```python
from build123d import *

# Parameters (mm, degrees)
F0_R      = 16.75
F1_DEPTH  = 6.2
F2_R      = 23.65
F3_DEPTH  = 2.2
F5_D      = 2
F6_R      = 16
F7_DEPTH  = 3.9
F8_R      = 12.5
F9_DEPTH  = 4.5
F11_D     = 1
F11_DEPTH = 4
F11_TIP   = 0.3004303095
F12_R     = 7.2
F13_DEPTH = 6.6
F15_D     = 3
F15_DEPTH = 1
F15_TIP   = 0.9012909285


with BuildPart() as f1:
    # F0 (on Top) → F1 (new body)
    with BuildSketch(Plane.XY):
        Circle(F0_R)
    extrude(amount=F1_DEPTH)

    # F2 (on face) → F3 (join)
    with BuildSketch(Plane.XY.offset(6.2)):
        Circle(F2_R)
    extrude(amount=F3_DEPTH)

    # F5 (through all)
    with Locations(Plane.XY.offset(8.4)):
        with Locations((0, 20.65), (17.8834245881, -10.325), (-17.8834245881, -10.325)):
            Hole(F5_D / 2)

    # F6 (on face) → F7 (join)
    with BuildSketch(Plane.XY.offset(8.4)):
        Circle(F6_R)
    extrude(amount=F7_DEPTH)

    # F8 (on face) → F9 (join)
    with BuildSketch(Plane.XY.offset(12.3)):
        Circle(F8_R)
    extrude(amount=F9_DEPTH)

    # F11
    with Locations(Plane.XY.offset(16.8)):
        with Locations((-8.6602540378, 5), (0, 10), (8.6602540378, 5), (8.6602540378, -5), (0, -10), (-8.6602540378, -5)):
            Hole(F11_D / 2, depth=F11_DEPTH)
            with Locations((0, 0, -(F11_DEPTH + F11_TIP / 2))):  # 118° drill point
                Cone(0, F11_D / 2, F11_TIP, mode=Mode.SUBTRACT)

    # F12 (on face) → F13 (join)
    with BuildSketch(Plane.XY.offset(16.8)):
        Circle(F12_R)
    extrude(amount=F13_DEPTH)

    # F15
    with Locations(Plane.XY.offset(23.4)):
        with Locations((0, 0)):
            Hole(F15_D / 2, depth=F15_DEPTH)
            with Locations((0, 0, -(F15_DEPTH + F15_TIP / 2))):  # 118° drill point
                Cone(0, F15_D / 2, F15_TIP, mode=Mode.SUBTRACT)


solid = f1.part
```
Design review of the part built by this model. Coordinates are the model's own, in mm. A direction names the side the tool comes from. Give positions to 0.01 mm unless a question says otherwise; leave off trailing zeros. Order: outer loops, then holes, each group sorted by start corner. A loop starts at its lowest first (then second) coordinate and runs counter-clockwise, first axis right, second up. Notation, with made-up numbers: (9, 86.25) - (42, 86.25) arc R26 ccw to (42, 125.25) - close; hole circle Ø10 at (21.5, 59.5). An arc over 180 degrees is marked (long way). Use a Markdown table: item, result. Add a question column.
(1) Add section D-D on y = -8.5. Give the boundary of the cut face in (x, z).
(2) Add section A-A on y = 20.65. Give the boundary of the cut face in (x, z), then the cut area to 3 significant figures.
(3) Mouldability with a two-part tool opening along X and no side actions: class faces 1 (the face through (0.13, 21.64, 7.28)), 2 (the face through (-5.127, -23.088, 7.285)), 3 (the face through (0, 0, 0)), 4 (the face through (-17.09, -10.933, 7.285)) as +X half, -X half, draft (parallel to the pull), parting line (faces both ways), or undercut.
(4) Wall thickness on probe 1 along X at (y, z) = (-5, 14.9); probe 2 along Y at (x, z) = (0, 11.25); probe 3 along Z at (x, y) = (15.5, 11): over which ranges is each line inside the solid? List them lowest first. Write a range as [from, to].
(5) Add section C-C on x = 14. Give the boundary of the cut face in (y, z), then the cut area to 3 significant figures.
(6) Machinability: for faces 5 (the face through (18.7, -10.9, 7.3)), 6 (the face through (-3.63, -16.35, 3.06)), 7 (the face through (4.9, -15.4, 8.4)), which of the approach directions +Z, -Z, +X, -X, +Y, -Y give a long, thin tool a straight path to every point of the face, cutting with its end or side? Answer none if there is none.
(7) Add section B-B on y = -3.5. Give the boundary of the cut face in (x, z).
(8) Clearance check with flat-ended pins moving along their axes: P1, Ø3, axis at x = 4.5, y = 16, coming from the +Z side; P2, Ø5, axis at y = -15, z = 17.5, coming from the +X side; P3, Ø12, axis at x = -3, z = 6, coming from the -Y side; P4, Ø2.5, axis at x = -17.88, y = -10.32, coming from the -Z side. State where each tip first meets the part, or that it passes through.
Report:
| question | item | result |
|---|---|---|
| 1 | outline | (-22.07, 6.2) - (-14.43, 6.2) - (-14.43, 0) - (14.43, 0) - (14.43, 6.2) - (22.07, 6.2) - (22.07, 8.4) - (13.56, 8.4) - (13.56, 12.3) - (9.17, 12.3) - (9.17, 16.8) - (-9.17, 16.8) - (-9.17, 12.3) - (-13.56, 12.3) - (-13.56, 8.4) - (-22.07, 8.4) - close |
| 2 | outline | (-11.53, 6.2) - (-1, 6.2) - (-1, 8.4) - (-11.53, 8.4) - close; (1, 6.2) - (11.53, 6.2) - (11.53, 8.4) - (1, 8.4) - close |
| 2 | area | 46.3 mm² |
| 3 | face 1 | undercut |
| 3 | face 2 | parting line |
| 3 | face 3 | draft |
| 3 | face 4 | undercut |
| 4 | probe 1 | x = [-11.46, -9.16], [-8.16, 8.16], [9.16, 11.46] |
| 4 | probe 2 | y = [-16, 16] |
| 4 | probe 3 | z = [6.2, 8.4] |
| 5 | outline | (-19.06, 6.2) - (-9.2, 6.2) - (-9.2, 0) - (9.2, 0) - (9.2, 6.2) - (19.06, 6.2) - (19.06, 8.4) - (7.75, 8.4) - (7.75, 12.3) - (-7.75, 12.3) - (-7.75, 8.4) - (-19.06, 8.4) - close |
| 5 | area | 258 mm² |
| 6 | face 5 | +Z, -Z |
| 6 | face 6 | -Z |
| 6 | face 7 | +Z |
| 7 | outline | (-23.39, 6.2) - (-16.38, 6.2) - (-16.38, 0) - (16.38, 0) - (16.38, 6.2) - (23.39, 6.2) - (23.39, 8.4) - (15.61, 8.4) - (15.61, 12.3) - (12, 12.3) - (12, 16.8) - (6.29, 16.8) - (6.29, 23.4) - (-6.29, 23.4) - (-6.29, 16.8) - (-12, 16.8) - (-12, 12.3) - (-15.61, 12.3) - (-15.61, 8.4) - (-23.39, 8.4) - close |
| 8 | P1 | stops at z = 12.3 |
| 8 | P2 | passes through |
| 8 | P3 | stops at y = -23.65 |
| 8 | P4 | stops at z = 6.2 |
